Source: three-view drawing plus pictorial views. Frame: mm from the lowest corner of the part. A direction names the side the tool comes from. Coordinates: 2 decimals unless noted, no trailing zeros. Write each loop counter-clockwise with the first axis right and the second up, starting at its lowest first coordinate (ties: lowest second). Pieces come first, ordered by that corner, then holes. Notation, with made-up numbers: M -30,-5 L 11,-5 A12 ccw 11,-1 Z; hole C -24,8 d8. An arc over 180 degrees is marked long. Write item = value, one per line. Start each with the question number.
Item 1: Pull-direction query (X, two-part tool) for the marked faces 3, 4 and 5; classes: +X half, -X half, draft (parallel to the pull), parting line (faces both ways), or undercut.
Item 2: Section B-B on x = 45. Output: boundary loops of the cut face in (y, z).
Item 3: First-contact query: pin 1 Ø12 at (x, z) = (60.5, 32.5) entering from -Y (1 decimal); pin 2 Ø21.5 at (x, y) = (52, 16) entering from +Z; pin 3 Ø5 at (x, y) = (69, 29) entering from +Z (1 decimal). Flat tips, straight axial feed; report the tip coordinate or a pass-through.
Item 4: Section C-C on z = 52.5. Output: boundary loops of the cut face in (x, y).
Item 5: Ray query, L1, parallel to X at y = 12, z = 25; L2, parallel to Z at x = 45.5, y = 7; L3, parallel to Y at x = 85, z = 31.5. Return the intervals inside material, ascending. Write a range as [from, to].
Item 6: Reachability of the marked faces 1 and 2 from +Z, -Z, +X, -X, +Y, -Y: full face, straight path, thin tool, end or side. Return the list, or none.
Item 7: Section A-A on y = 22. Output: boundary loops of the cut face in (x, z).
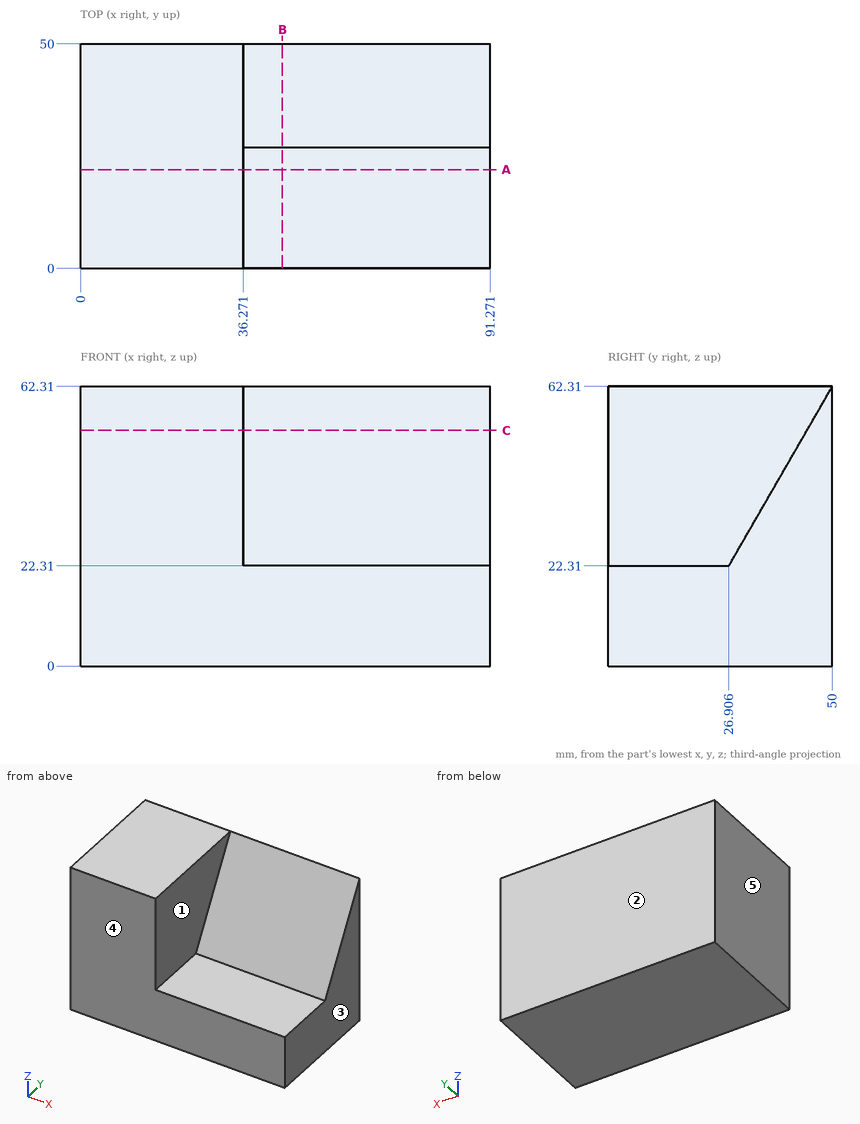
Responses:
q1.face_3 = +X half
q1.face_4 = draft
q1.face_5 = -X half
q2.outline = M 0,0 L 50,0 L 50,62.31 L 26.91,22.31 L 0,22.31 Z
q3.pin_1 = 29.3
q3.pin_2 = 22.31
q3.pin_3 = 30.3
q4.outline = M 0,0 L 36.27,0 L 36.27,44.34 L 91.27,44.34 L 91.27,50 L 0,50 Z
q5.L1 = [0, 36.27]
q5.L2 = [0, 22.31]
q5.L3 = [32.21, 50]
q6.face_1 = +Z, +X, -Y
q6.face_2 = +Z, -Z, +X, -X, +Y
q7.outline = M 0,0 L 91.27,0 L 91.27,22.31 L 36.27,22.31 L 36.27,62.31 L 0,62.31 Z
